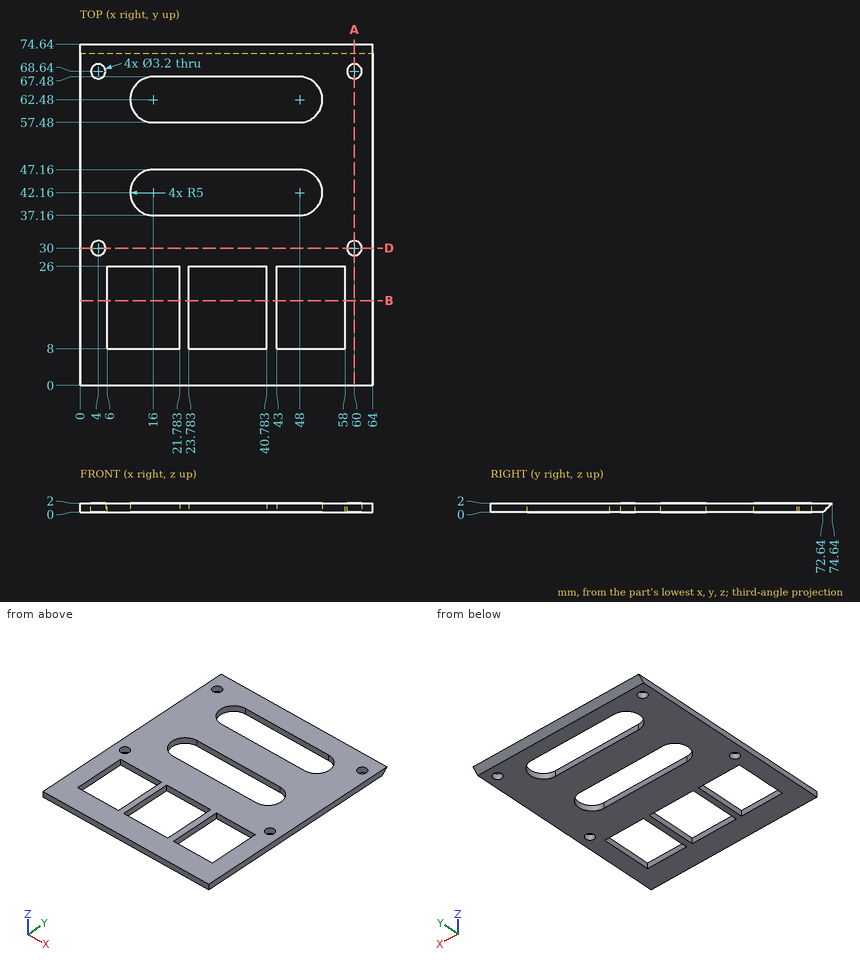
The figure shows three views and two pictorial views of one solid part (mm, origin at its lowest corner). Answer the questions. Give positions to 0.01 mm unless a question says otherwise; leave off trailing zeros. Loops run counter-clockwise (first coordinate to the right, second up) from the corner with the lowest first, then second, coordinate; pieces in that order, holes last. Notation, with made-up numbers: M 65.25,-36 L 85.25,-36 A17 cw 85.25,-6 Z; hole C -30.5,-17 d8. An arc over 180 degrees is marked long. Write each question's results on one line, items separated by ' | '.
1. Section B-B on y = 18.5 is taken. Give the vertices of the cut face in (x, z).
Values:
outline: M 0,0 L 6,0 L 6,2 L 0,2 Z; M 21.78,0 L 23.78,0 L 23.78,2 L 21.78,2 Z; M 40.78,0 L 43,0 L 43,2 L 40.78,2 Z; M 58,0 L 64,0 L 64,2 L 58,2 Z
2. Straight lines are drawn through the part: line 1 (X direction, y = 68.64, z = 0.5); line 2 (X direction, y = 16.5, z = 1.45); line 3 (Y direction, x = 4, z = 0.9). For each, find the intervals that lie inside material, in ascending order. Write a range as [from, to].
Values:
line 1: x = [0, 2.4], [5.6, 58.4], [61.6, 64] | line 2: x = [0, 6], [21.78, 23.78], [40.78, 43], [58, 64] | line 3: y = [0, 28.4], [31.6, 67.04], [70.24, 73.54]
3. Section D-D on y = 30 is taken. Give the vertices of the cut face in (x, z).
Values:
outline: M 0,0 L 2.4,0 L 2.4,2 L 0,2 Z; M 5.6,0 L 58.4,0 L 58.4,2 L 5.6,2 Z; M 61.6,0 L 64,0 L 64,2 L 61.6,2 Z
4. Given pin 1 (1 mm diameter, centred on x = 32.5, z = 1, fed in from +Y); pin 2 (1 mm diameter, centred on x = 53, z = 1.5, fed in from -Y); pin 3 (1 mm diameter, centred on x = 51.5, z = 0.5, fed in from +Y), each flat-ended and moving along its own axis, determine where each tip first touches the part or whether it passes through.
Values:
pin 1: stops at y = 74.14 | pin 2: stops at y = 0 | pin 3: stops at y = 73.64
5. Section A-A on x = 60 is taken. State how many separate pieces and enclosed holes the cut face has.
Values:
separate pieces: 3 | enclosed holes: 0
